Part model, mm, in its own coordinate system. Coordinates: 2 decimals unless noted, no trailing zeros. Order: outer loops, then holes, each group sorted by start corner. A loop starts at its lowest first (then second) coordinate and runs counter-clockwise, first axis right, second up. Notation, with made-up numbers: M -15.75,-26 L 43.25,-26 A32 cw 43.25,13 Z; hole C 27.25,33 d3. An arc over 180 degrees is marked long. Answer in a Markdown table with one row per item. Add a question column.
from build123d import *

# Parameters (mm, degrees)
SKETCH1_R           = 34.13125
BOSS_EXTRUDE1_DEPTH = 1.59
SKETCH2_R           = 0.75
CUT_EXTRUDE1_DEPTH  = 1.59
SKETCH3_R           = 1.5
CUT_EXTRUDE2_DEPTH  = 1.59


with BuildPart() as part:
    # Sketch1 → Boss-Extrude1 (new body)
    with BuildSketch(Plane(origin=(0, 0, 0), x_dir=(1, 0, 0), z_dir=(0, 1, 0))):
        with Locations(Location((0, 0, 0), (0, 0, 90))):
            Circle(SKETCH1_R)
    extrude(amount=BOSS_EXTRUDE1_DEPTH)

    # Sketch2 → Cut-Extrude1 (cut)
    with BuildSketch(Plane(origin=(0, 1.59, 0), x_dir=(1, 0, 0), z_dir=(0, 1, 0))):
        with Locations(Location((0, -7.5, 0), (0, 0, 270))):
            Circle(SKETCH2_R)
        with Locations(Location((0, 7.5, 0), (0, 0, 270))):
            Circle(SKETCH2_R)
        with Locations(Location((-7.5, 0, 0), (0, 0, 270))):
            Circle(SKETCH2_R)
        with Locations(Location((7.5, 0, 0), (0, 0, 270))):
            Circle(SKETCH2_R)
    extrude(amount=-CUT_EXTRUDE1_DEPTH, mode=Mode.SUBTRACT)

    # Sketch3 → Cut-Extrude2 (cut)
    with BuildSketch(Plane(origin=(0, 1.59, 0), x_dir=(1, 0, 0), z_dir=(0, 1, 0))):
        with Locations(Location((-15.909, 15.910805102, 0), (0, 0, 270))):
            Circle(SKETCH3_R)
        with Locations(Location((15.910805102, 15.909, 0), (0, 0, 270))):
            Circle(SKETCH3_R)
        with Locations(Location((15.909, -15.910805102, 0), (0, 0, 270))):
            Circle(SKETCH3_R)
        with Locations(Location((-15.910805102, -15.909, 0), (0, 0, 270))):
            Circle(SKETCH3_R)
    extrude(amount=-CUT_EXTRUDE2_DEPTH, mode=Mode.SUBTRACT)


solid = part.part
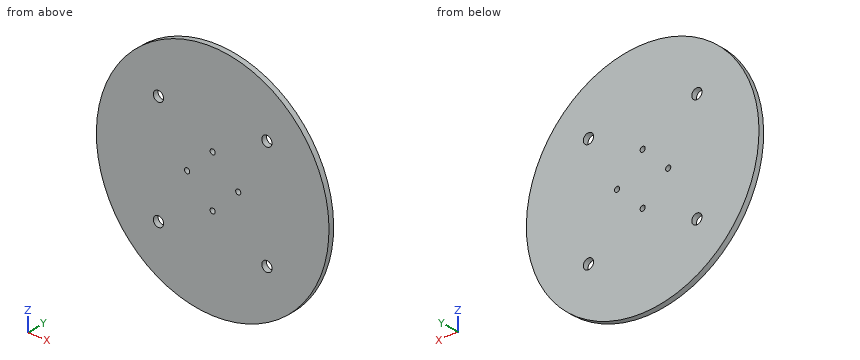
(1) Slice it at B-B (y = 0.7). State how many separate pieces and enclosed holes the cut face has, and give its area (3 significant figures).
(2) Wall check: line 1 (X direction, y = 0.45, z = 0); line 2 (Z direction, x = -8, y = 0.55); line 3 (X direction, y = 0.6, z = 7.5). Give the ranges that are in metal, low to high.
(3) Slice it at A-A (z = -16.5). List the corners of the cut face in (x, y).
(4) Slice it at D-D (z = 12). List the corners of the cut face in (x, y), and give its area (3 significant figures).
(5) Slice it at C-C (x = 30.5). List the corners of the cut face in (y, z), and give its area (3 significant figures).
Computed:
| question | item | result |
|---|---|---|
| 1 | separate pieces | 1 |
| 1 | enclosed holes | 8 |
| 1 | area | 3,620 mm^2 |
| 2 | line 1 | x = -34.13 to -8.25, -6.75 to 6.75, 8.25 to 34.13 |
| 2 | line 2 | z = -33.18 to -0.56, 0.56 to 33.18 |
| 2 | line 3 | x = -33.3 to -0.75, 0.75 to 33.3 |
| 3 | outline | M -29.88,0 L -17.29,0 L -17.29,1.59 L -29.88,1.59 Z; M -14.53,0 L 14.53,0 L 14.53,1.59 L -14.53,1.59 Z; M 17.29,0 L 29.88,0 L 29.88,1.59 L 17.29,1.59 Z |
| 4 | outline | M -31.95,0 L 31.95,0 L 31.95,1.59 L -31.95,1.59 Z |
| 4 | area | 102 mm^2 |
| 5 | outline | M 0,-15.32 L 1.59,-15.32 L 1.59,15.32 L 0,15.32 Z |
| 5 | area | 48.7 mm^2 |
